from build123d import *

# Parameters (mm, degrees)
HEX_DIE_START = -1e-06
SKETCH2_R     = 7.580831409
HEX_DIE_DEPTH = 6.000001
SKETCH4_R     = 5.6875
INDENT_DEPTH  = 0.75


with BuildPart() as part:
    # BodySke → Base-Revolve (revolve)
    with BuildSketch(Plane.XY, mode=Mode.PRIVATE) as base_revolve_sk:
        Polygon((6, 4), (6, 7.505773672), (0.5806837, 7.505773672), (0, 6.5), (0, 0), (22, 0), (22, 4), align=None)
    revolve(base_revolve_sk.sketch.rotate(Axis((-25.4, 0, 0), (1, 0, 0)), 90), axis=Axis((-25.4, 0, 0), (1, 0, 0)))

    # Sketch2 → Hex-Die (cut)
    with BuildSketch(Plane(origin=(0, 0, 0), x_dir=(0, 0, -1), z_dir=(1, 0, 0)).offset(HEX_DIE_START)):
        Circle(SKETCH2_R)
        Polygon((-6.5, 3.752776766), (0, 7.505553532), (6.5, 3.752776766), (6.5, -3.752776766), (0, -7.505553532), (-6.5, -3.752776766), align=None, mode=Mode.SUBTRACT)
    extrude(amount=HEX_DIE_DEPTH, mode=Mode.SUBTRACT)

    # Sketch4 → Indent (cut)
    with BuildSketch(Plane(origin=(0, 0, 0), x_dir=(0, 0, -1), z_dir=(1, 0, 0))):
        Circle(SKETCH4_R)
    extrude(amount=INDENT_DEPTH, mode=Mode.SUBTRACT)


solid = part.part
Read the model definition and answer for the solid it produces. Units are mm, in the model's axes. A direction names the side the tool comes from. Coordinates: 2 decimals unless noted, no trailing zeros. Write each loop counter-clockwise with the first axis right and the second up, starting at its lowest first coordinate (ties: lowest second). Pieces come first, ordered by that corner, then holes. Notation, with made-up numbers: M -14.5,-31.5 L 10.5,-31.5 A19 ccw 10.5,-4.5 Z; hole C -27,42 d5. An arc over 180 degrees is marked long. Use a Markdown table: item, result.
Q1. Which of the six approach directions +Z, -Z, +X, -X, +Y, -Y give full straight-line access (tool end or side, diameter ignored) to faces 5 (the face through (6, 3, -3)), 6 (the face through (2.96, 5.66, -3.2))?
Answer block:
| item | result |
|---|---|
| face 5 | +X |
| face 6 | -Z, +X, -X, +Y |
Q2. The part is cut by section A-A, the plane x = 10. Write down the section's boundary in (y, z).
Answer block:
| item | result |
|---|---|
| outline | C 0,0 d8 |
Q3. Determine the mould class of faces 1 (the face through (0.138, 3.356, -5.845)), 2 (the face through (0.37, -3.461, 4.513)), 3 (the face through (0.75, 0, 0)), 4 (the face through (22, 0, 0)) for opening direction Z: released by +Z, released by -Z, zero draft, split by the parting line, or undercut.
Answer block:
| item | result |
|---|---|
| face 1 | released by -Z |
| face 2 | undercut |
| face 3 | undercut |
| face 4 | zero draft |
Q4. Each of these flat-tipped pins is pushed along its axis until it touches: pin 1 Ø3 at (x, y) = (12, 1.5) entering from +Z; pin 2 Ø3 at (x, z) = (16, 3.5) entering from +Y; pin 3 Ø1 at (x, y) = (15, -2) entering from +Z; pin 4 Ø2 at (y, z) = (2.5, -5) entering from -X. Where does it stop, or does it pass through?
Answer block:
| item | result |
|---|---|
| pin 1 | stops at z = 4 |
| pin 2 | stops at y = 3.46 |
| pin 3 | stops at z = 3.71 |
| pin 4 | stops at x = 0 |
Q5. Straight lines are drawn through the part: L1, parallel to X at y = 3, z = 5; L2, parallel to X at y = -1.25, z = 0.5; L3, parallel to Y at x = 0.55, z = 0. For each, find the intervals that lie inside material, in ascending order. Write a range as [from, to].
Answer block:
| item | result |
|---|---|
| L1 | x = [0, 6] |
| L2 | x = [0.75, 22] |
| L3 | y = [-7.45, -5.69], [5.69, 7.45] |
